from build123d import *

# Parameters (mm, degrees)
F0_R     = 4.5
F1_DEPTH = 18.8087
F2_W     = 10.2
F2_H     = 10.2
F3_DEPTH = 10
F4_R     = 2.36
F5_DEPTH = 12.75
F7_DEPTH = 12.75


with BuildPart() as f1:
    # F0 (on Top) → F1 (new body)
    with BuildSketch(Plane.XY):
        Circle(F0_R)
    extrude(amount=F1_DEPTH)

    # F2 (on face) → F3 (join)
    with BuildSketch(Plane.XY.offset(18.8087)):
        Rectangle(F2_W, F2_H)
    extrude(amount=F3_DEPTH)

    # F4 (on face) → F5 (join)
    with BuildSketch(Plane.XY.offset(28.8087)):
        Circle(F4_R)
    extrude(amount=F5_DEPTH)

    # F6 (on face) → F7 (cut)
    with BuildSketch(Plane.XY.offset(41.5587)):
        with BuildLine():
            ThreePointArc((-1.538018, -1.79), (-0.820122, -2.212917), (0, -2.36))
            Line((0, -2.36), (0, -1.79))
            Line((0, -1.79), (-1.538018, -1.79))
        make_face()
        with BuildLine():
            Line((0, -1.79), (0, -2.36))
            ThreePointArc((0, -2.36), (0.820122, -2.212917), (1.538018, -1.79))
            Line((1.538018, -1.79), (0, -1.79))
        make_face()
    extrude(amount=-F7_DEPTH, mode=Mode.SUBTRACT)


solid = f1.part
Verification items for the finished model (mm, model axes). A direction names the side the tool comes from. Round coordinates to 2 decimals unless told otherwise and drop trailing zeros. Loops run counter-clockwise (first coordinate to the right, second up) from the corner with the lowest first, then second, coordinate; pieces in that order, holes last. Notation, with made-up numbers: M 32.5,-10 L 55.5,-10 A8 cw 55.5,-5 Z; hole C 30,65 d2. An arc over 180 degrees is marked long. Write each question's results on one line, items separated by ' | '.
1) Section check D-D on y = 3.25. Record the boundary of the cut face in (x, z), then the cut area to 3 significant figures.
Checks:
outline: M -5.1,18.81 L -3.11,18.81 L -3.11,0 L 3.11,0 L 3.11,18.81 L 5.1,18.81 L 5.1,28.81 L -5.1,28.81 Z | area: 219 mm2
2) Access from +Z, -Z, +X, -X, +Y, -Y to the whole of each face (thin tool, end or side, straight path). Record for faces 1 (the flat face through (0, -5.1, 24)), 2 (the cylindrical face through (0.08, 2.36, 35.09)), 3 (the flat face through (0, -1.79, 35)), 4 (the flat face through (-1.2, 4.6, 18.809)), 5 (the flat face through (0, 0, 0)).
Checks:
face 1: +Z, -Z, +X, -X, -Y | face 2: +Z | face 3: +Z, +X, -X, -Y | face 4: -Z | face 5: -Z, +X, -X, +Y, -Y
3) Section check C-C on z = 37. Record the boundary of the cut face in (x, y), then the cut area to 3 significant figures.
Checks:
outline: M -1.54,-1.79 L 1.54,-1.79 A2.36 ccw long Z | area: 16.3 mm2
4) Section check A-A on y = 0. Record the boundary of the cut face in (x, z), then the cut area to 3 significant figures.
Checks:
outline: M -5.1,18.81 L -4.5,18.81 L -4.5,0 L 4.5,0 L 4.5,18.81 L 5.1,18.81 L 5.1,28.81 L 2.36,28.81 L 2.36,41.56 L -2.36,41.56 L -2.36,28.81 L -5.1,28.81 Z | area: 331 mm2
5) Section check B-B on x = 0. Record the boundary of the cut face in (y, z).
Checks:
outline: M -5.1,18.81 L -4.5,18.81 L -4.5,0 L 4.5,0 L 4.5,18.81 L 5.1,18.81 L 5.1,28.81 L 2.36,28.81 L 2.36,41.56 L -1.79,41.56 L -1.79,28.81 L -5.1,28.81 Z
6) Scan lines: L1, parallel to Z at x = 3.25, y = -4.5; L2, parallel to Z at x = 3.5, y = 2; L3, parallel to X at y = -0.5, z = 12. Record each from-to range of solid material in increasing order. Write a range as from..to.
Checks:
L1: z = 18.81..28.81 | L2: z = 0..28.81 | L3: x = -4.47..4.47
7) Gauge pin test, flat ends, axial feed: P1, Ø3, axis at x = 2, y = -2, coming from the +Z side; P2, Ø4, axis at y = -1, z = 34.5, coming from the -X side; P3, Ø0.9, axis at x = -0.5, z = 36, coming from the -Y side. Record the tip position at first contact, or that the pin passes through.
Checks:
P1: stops at z = 41.56 | P2: stops at x = -2.36 | P3: stops at y = -1.79
